```python
from build123d import *

# Parameters (mm, degrees)
F1_DEPTH = 100
F2_R     = 5
F4_D     = 60
F6_D     = 10


with BuildPart() as f1:
    # F0 (on Front) → F1 (new body)
    with BuildSketch(Plane.XZ):
        Polygon((-109.5206329271, 0), (-104.5206329271, 0), (-104.5206329271, 99.8773593255), (75.4793670729, 99.8773593255), (75.4793670729, 0), (80.4793670729, 0), (80.4793670729, 104.8773593255), (-109.5206329271, 104.8773593255), align=None)
    extrude(amount=F1_DEPTH)

    # F2
    f2_edges = [f1.edges().sort_by_distance(p)[0] for p in [
        (80.479367, -50, 104.877359),
        (-109.520633, -50, 104.877359),
    ]]
    fillet(f2_edges, radius=F2_R)

    # F4 (through all)
    with Locations(Plane(origin=(0, 0, 0), x_dir=(1, 0, 0), z_dir=(0, 0, -1))):
        with Locations((-14.5206329271, 50)):
            Hole(F4_D / 2)

    # F6 (through all)
    with Locations(Plane(origin=(0, 0, 0), x_dir=(1, 0, 0), z_dir=(0, 0, -1))):
        with Locations((-49.5206329271, 15), (20.4793670729, 15), (20.4793670729, 85), (-49.5206329271, 85)):
            Hole(F6_D / 2)


solid = f1.part
```
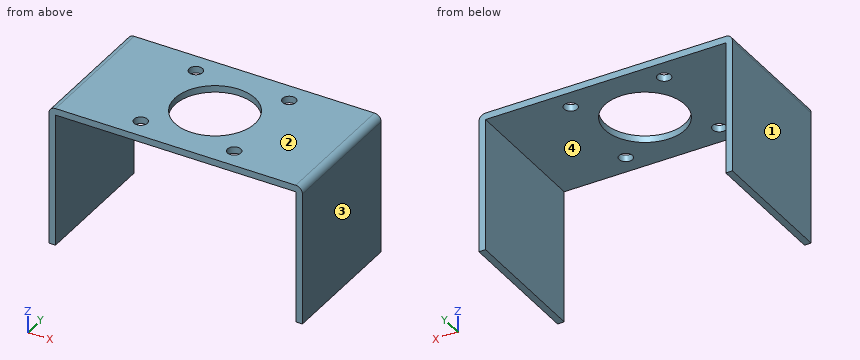
CAD build for the part. Positions are in the model's coordinates, mm. Face numbers are marked on the shaded views. Round coordinates to 2 decimals unless told otherwise and drop trailing zeros. Write each loop counter-clockwise with the first axis right and the second up, starting at its lowest first coordinate (ties: lowest second). Pieces come first, ordered by that corner, then holes. Notation, with made-up numbers: (14.25, 58) - (27.25, 58) arc R9 ccw to (27.25, 72) - close; hole circle Ø10 at (82, 63.5). An arc over 180 degrees is marked (long way). Write item = value, one per line. Start each with the question number.
Q1. Band-saw the part on D-D (x = -25). Give the cut face in (y, z), then the cut area to 3 significant figures.
Q2. Mould opens along X. For the marked faces 1, 2, 3 and 4 say: pulls with the +X half, pulls with the -X half, needs draft (parallel to the pull), parting line crosses it, or undercut.
Q3. Probe L1, parallel to X at y = -43, z = 6; L2, parallel to X at y = -85, z = 103.8; L3, parallel to Z at x = -31, y = -87.5. List the from-to ranges inside material, lowest first. Write a range as from..to.
Q4. Band-saw the part on B-B (z = 87.5). Give the cut face in (x, y).
Q5. Band-saw the part on A-A (y = -15). Give the cut face in (x, z).
Q6. Band-saw the part on C-C (y = -50). Give the cut face in (x, z).
Q7. Drop flat-ended pins along their axis: pin 1 (11.5 mm diameter, centred on x = -49.52, y = -85, fed in from -Z); pin 2 (9 mm diameter, centred on x = -49.52, y = -15, fed in from -Z); pin 3 (11.5 mm diameter, centred on x = 20.48, y = -85, fed in from +Z). Give the stop position or say it passes through.
Answers below:
q1.outline = (-100, 99.88) - (-78.11, 99.88) - (-78.11, 104.88) - (-100, 104.88) - close; (-21.89, 99.88) - (0, 99.88) - (0, 104.88) - (-21.89, 104.88) - close
q1.area = 219 mm2
q2.face_1 = pulls with the -X half
q2.face_2 = needs draft
q2.face_3 = pulls with the +X half
q2.face_4 = undercut
q3.L1 = -109.52..-104.52, 75.48..80.48
q3.L2 = -107.62..-54.52, -44.52..15.48, 25.48..78.58
q3.L3 = 99.88..104.88
q4.outline = (-109.52, -100) - (-104.52, -100) - (-104.52, 0) - (-109.52, 0) - close; (75.48, -100) - (80.48, -100) - (80.48, 0) - (75.48, 0) - close
q5.outline = (-109.52, 0) - (-104.52, 0) - (-104.52, 99.88) - (-54.52, 99.88) - (-54.52, 104.88) - (-104.52, 104.88) arc R5 ccw to (-109.52, 99.88) - close; (-44.52, 99.88) - (15.48, 99.88) - (15.48, 104.88) - (-44.52, 104.88) - close; (25.48, 99.88) - (75.48, 99.88) - (75.48, 0) - (80.48, 0) - (80.48, 99.88) arc R5 ccw to (75.48, 104.88) - (25.48, 104.88) - close
q6.outline = (-109.52, 0) - (-104.52, 0) - (-104.52, 99.88) - (-44.52, 99.88) - (-44.52, 104.88) - (-104.52, 104.88) arc R5 ccw to (-109.52, 99.88) - close; (15.48, 99.88) - (75.48, 99.88) - (75.48, 0) - (80.48, 0) - (80.48, 99.88) arc R5 ccw to (75.48, 104.88) - (15.48, 104.88) - close
q7.pin_1 = 99.88
q7.pin_2 = through
q7.pin_3 = 104.88
